Read the model definition and answer for the solid it produces. Units are mm, in the model's axes. A direction names the side the tool comes from. Coordinates: 2 decimals unless noted, no trailing zeros. Order: outer loops, then holes, each group sorted by start corner. A loop starts at its lowest first (then second) coordinate and runs counter-clockwise, first axis right, second up. Notation, with made-up numbers: (63, 69) -> (95, 69) arc R17 ccw to (95, 98) -> close; hole circle Ø11 at (43.25, 83). An arc over 180 degrees is marked (long way). Answer in a Markdown table with one row per item.
Autodesk Inventor part; units mm, degrees
ref_plane "YZ Plane" through (0, 0, 0) normal (1, 0, 0) x (0, 1, 0)
ref_plane "XZ Plane" through (0, 0, 0) normal (0, 1, 0) x (-1, 0, 0)
ref_plane "XY Plane" through (0, 0, 0) normal (0, 0, 1) x (1, 0, 0)
sketch "Sketch5" plane through (0, 0, 0) normal (1, 0, 0) x (0, 1, 0)
  line L0 (0, 0) -> (101.6, 0)
  line L1 (101.6, 0) -> (101.6, -20.32)
  line L2 (101.6, -20.32) -> (0, -20.32)
  line L3 (0, -20.32) -> (0, 0)
  line L4 (101.6, -6.35) -> (6.35, -6.35)
  line L5 (6.35, -6.35) -> (6.35, -13.97)
  line L6 (6.35, -13.97) -> (101.6, -13.97)
  line L7 (101.6, -13.97) -> (101.6, -6.35)
  line L8 (101.6, 0) -> (50.8, 0)
  line L9 (50.8, -6.35) -> (101.6, -6.35)
  line L10 (101.6, -6.35) -> (101.6, 0)
  dimension "d26" = 101.6
  dimension "d27" = 20.32
  dimension "d28" = 95.25
  dimension "d29" = 7.62
  dimension "d30" = 6.35
  dimension "d31" = 50.8
extrude "Extrusion4" add sketch "Sketch5" against normal blind 228.6
sketch "Sketch6" plane through (0, 0, 0) normal (1, 0, 0) x (0, 0, -1)
  line L0 (0, 101.6) -> (0, 0)
  line L1 (20.32, 0) -> (20.32, 101.6)
  line L2 (20.32, 101.6) -> (0, 101.6)
  line L3 (0, 0) -> (20.32, 0)
  line L4 (0, 101.6) -> (20.32, 101.6)
  line L5 (13.97, 101.6) -> (6.35, 101.6)
  line L6 (6.35, 101.6) -> (6.35, 6.35)
  line L7 (6.35, 6.35) -> (13.97, 6.35)
  line L8 (13.97, 6.35) -> (13.97, 101.6)
  line L9 (0, 0) -> (0, 101.6)
  line L10 (0, 101.6) -> (6.35, 101.6)
  line L11 (6.35, 101.6) -> (6.35, 50.8)
  line L12 (6.35, 50.8) -> (0, 50.8)
  line L13 (0, 50.8) -> (0, 101.6)
  dimension "d34" = 7.62
  dimension "d35" = 95.25
  dimension "d36" = 6.35
  dimension "d37" = 50.8
extrude "Extrusion5" cut sketch "Sketch6" against normal blind 228.6 contours L2 L8 L7 L6
sketch "Sketch7" plane through (0, 0, 0) normal (1, 0, 0) x (0, 0, -1)
  line L0 (6.35, 6.35) -> (6.35, 101.6)
  line L1 (6.35, 101.6) -> (0, 101.6)
  line L2 (0, 101.6) -> (0, 0)
  line L3 (0, 0) -> (20.32, 0)
  line L4 (20.32, 0) -> (20.32, 101.6)
  line L5 (20.32, 101.6) -> (13.97, 101.6)
  line L6 (13.97, 101.6) -> (13.97, 6.35)
  line L7 (13.97, 6.35) -> (6.35, 6.35)
  line L8 (0, 101.6) -> (0, 0)
  line L9 (6.35, 6.35) -> (6.35, 101.6)
  line L10 (0, 101.6) -> (3.175, 101.6)
  line L11 (6.35, 98.425) -> (6.35, 50.8)
  line L12 (6.35, 50.8) -> (0, 50.8)
  line L13 (0, 50.8) -> (0, 101.6)
  arc A0 (6.35, 98.425) -> (3.175, 101.6) centre (3.175, 98.425) ccw
  line L14 (0, 0) -> (20.32, 0)
  line L15 (0, 50.8) -> (3.175, 50.8)
  line L16 (6.35, 47.625) -> (6.35, 0)
  line L17 (6.35, 0) -> (0, 0)
  line L18 (0, 0) -> (0, 50.8)
  arc A1 (6.35, 47.625) -> (3.175, 50.8) centre (3.175, 47.625) ccw
  line L19 (6.35, 50.8) -> (6.35, 41.6275)
  dimension "d40" = 50.8
  dimension "d47" = 3.175
  dimension "d48" = 3.175
extrude "Extrusion6" cut sketch "Sketch7" against normal blind 228.6 contours A1 L12 L0 | L12 L2 L1 A0 L0 | A0 L1 L0
sketch "Sketch8" plane through (0, 50.8, 0) normal (0, 1, 0) x (1, 0, 0)
  line L0 (0, 13.97) -> (0, 6.35)
  line L1 (0, 13.97) -> (-228.6, 13.97)
  line L2 (-228.6, 6.35) -> (-228.6, 13.97)
  line L3 (0, 6.35) -> (-228.6, 6.35)
  line L4 (0, 3.175) -> (0, 0)
  line L5 (-228.6, 0) -> (-228.6, 3.175)
  line L6 (0, 0) -> (-228.6, 0)
  line L7 (-228.6, 13.97) -> (0, 13.97)
  line L8 (0, 20.32) -> (0, 13.97)
  line L9 (0, 20.32) -> (-228.6, 20.32)
  line L10 (-228.6, 13.97) -> (-228.6, 20.32)
  line L11 (-228.6, 13.97) -> (0, 13.97)
  line L12 (0, 0) -> (-228.6, 0)
  line L13 (0, 13.97) -> (-228.6, 13.97)
  line L14 (-107.95, 0) -> (-120.65, 0)
  line L15 (-120.65, 0) -> (-120.65, 13.97)
  line L16 (-120.65, 13.97) -> (-107.95, 13.97)
  line L17 (-107.95, 13.97) -> (-107.95, 0)
  line L18 (0, 3.175) -> (-228.6, 3.175)
  dimension "d43" = 12.7
  dimension "d44" = 107.95
extrude "Extrusion7" cut sketch "Sketch8" against normal blind 228.6 contours L17 L3 L15 L1 | L17 L18 L15 L3 | L17 L6 L15 L18
properties part number "Handles"
Q1. For a pull along X with two mould halves and no side action, classify faces 1 (the face through (0, 39, -15)), 2 (the face through (-107.95, 26, -4)), 3 (the face through (-113, 0, -15)) as pulls with the +X half, pulls with the -X half, needs draft (parallel to the pull), parting line crosses it, or undercut.
Outcome:
| item | result |
|---|---|
| face 1 | pulls with the +X half |
| face 2 | undercut |
| face 3 | needs draft |
Q2. Given pin 1 (6 mm diameter, centred on x = -94.5, y = 73, fed in from +Z); pin 2 (1 mm diameter, centred on x = -162.5, z = -2, fed in from +Y); pin 3 (2.5 mm diameter, centred on x = -198.5, z = -10, fed in from +Y), each flat-ended and moving along its own axis, determine where each tip first touches the part or whether it passes through.
Outcome:
| item | result |
|---|---|
| pin 1 | z = -13.97 |
| pin 2 | y = 50.8 |
| pin 3 | y = 6.35 |
Q3. The part is cut by section B-B (x = -194.5). Write down the section's boundary in (y, z) (3 decimals).
Outcome:
| item | result |
|---|---|
| outline | (0, -20.32) -> (101.6, -20.32) -> (101.6, -13.97) -> (6.35, -13.97) -> (6.35, -6.35) -> (47.625, -6.35) arc R3.175 ccw to (50.8, -3.175) -> (50.8, 0) -> (0, 0) -> close |
Q4. For faces 4 (the face through (-53, 27, -6.35)), 5 (the face through (-174, 25, 0)), 6 (the face through (-120.65, 26, -4)), determine the directions among +Z, -Z, +X, -X, +Y, -Y from which every point of the face is accessible in a straight line to the end or side of a thin tool.
Outcome:
| item | result |
|---|---|
| face 4 | +X, -X, +Y |
| face 5 | +Z, +X, -X, +Y, -Y |
| face 6 | +Z, +Y, -Y |
Q5. The part is cut by section C-C (y = 73.5). Write down the section's boundary in (x, z), then the cut area to 3 significant figures.
Outcome:
| item | result |
|---|---|
| outline | (-228.6, -20.32) -> (0, -20.32) -> (0, -13.97) -> (-228.6, -13.97) -> close |
| area | 1,450 mm² |
Q6. The part is cut by section A-A (y = 40). Write down the section's boundary in (x, z), then the cut area to 3 significant figures.
Outcome:
| item | result |
|---|---|
| outline | (-228.6, -20.32) -> (0, -20.32) -> (0, -13.97) -> (-228.6, -13.97) -> close; (-228.6, -6.35) -> (-120.65, -6.35) -> (-120.65, 0) -> (-228.6, 0) -> close; (-107.95, -6.35) -> (0, -6.35) -> (0, 0) -> (-107.95, 0) -> close |
| area | 2,820 mm² |
Q7. Consider line 1 (Z direction, x = -27, y = 39); line 2 (Y direction, x = -36.5, z = -9); line 3 (Z direction, x = -23, y = 95). Determine where each line is inside the solid, lowest interval first.
Outcome:
| item | result |
|---|---|
| line 1 | -20.32 to -13.97, -6.35 to 0 |
| line 2 | 0 to 6.35 |
| line 3 | -20.32 to -13.97 |
